```python
from build123d import *

# Parameters (mm, degrees)
ESQUISSE1_R        = 3.25
ESQUISSE1_R_2      = 2
BOSS_EXTRU_1_DEPTH = 1.5
ESQUISSE2_W        = 10
ESQUISSE2_H        = 1.5
BOSS_EXTRU_2_DEPTH = 6
CONG_1_START       = -20
CONG_1_DEPTH       = 10
CONG_1_START_2     = -6
CONG_1_2_DEPTH     = 1.5
CONG_1_START_3     = -24.5
CONG_1_3_DEPTH     = 29


with BuildPart() as part:
    # Esquisse1 → Boss.-Extru.1 (new body)
    with BuildSketch(Plane.XY):
        with BuildLine():
            Line((0, -4.5), (-20, -4.5))
            ThreePointArc((-20, -4.5), (-24.5, 0), (-20, 4.5))
            Line((-20, 4.5), (0, 4.5))
            ThreePointArc((0, 4.5), (4.5, 0), (0, -4.5))
        make_face()
        Circle(ESQUISSE1_R, mode=Mode.SUBTRACT)
        with Locations((-20, 0)):
            Circle(ESQUISSE1_R_2, mode=Mode.SUBTRACT)
    extrude(amount=BOSS_EXTRU_1_DEPTH)

    # Esquisse2 → Boss.-Extru.2 (add)
    with BuildSketch(Plane.XY.offset(1.5)):
        with Locations((-15, -5.25)):
            Rectangle(ESQUISSE2_W, ESQUISSE2_H)
    extrude(amount=-BOSS_EXTRU_2_DEPTH)

    # Congé1: read off the stored shape, not the designer's step
    # Congé1 outline → Congé1 (add)
    with BuildSketch(Plane.YZ.offset(CONG_1_START)):
        with BuildLine():
            ThreePointArc((-4.5, -1.5), (-4.060660172, -0.439339828), (-3, 0))
            Line((-3, 0), (-4.5, 0))
            Line((-4.5, 0), (-4.5, -1.5))
        make_face()
    extrude(amount=CONG_1_DEPTH)

    # Cong_1 2 outline → Cong_1 2 (cut)
    with BuildSketch(Plane(origin=(0, 0, 0), x_dir=(1, 0, 0), z_dir=(0, 1, 0)).offset(CONG_1_START_2)):
        with BuildLine():
            ThreePointArc((-20, 3.5), (-19.707106781, 4.207106781), (-19, 4.5))
            Line((-19, 4.5), (-20, 4.5))
            Line((-20, 4.5), (-20, 3.5))
        make_face()
        with BuildLine():
            ThreePointArc((-11, 4.5), (-10.292893219, 4.207106781), (-10, 3.5))
            Line((-10, 3.5), (-10, 4.5))
            Line((-10, 4.5), (-11, 4.5))
        make_face()
    extrude(amount=CONG_1_2_DEPTH, mode=Mode.SUBTRACT)

    # Cong_1 3 outline → Cong_1 3 (cut)
    with BuildSketch(Plane.YZ.offset(CONG_1_START_3)):
        with BuildLine():
            ThreePointArc((-6, -1.5), (-5.121320344, 0.621320344), (-3, 1.5))
            Line((-3, 1.5), (-6, 1.5))
            Line((-6, 1.5), (-6, -1.5))
        make_face()
    extrude(amount=CONG_1_3_DEPTH, mode=Mode.SUBTRACT)


solid = part.part
```
Source: CAD feature listing. Evaluate the final solid. Frame: model axes, mm. A direction names the side the tool comes from. Coordinates: 2 decimals unless noted, no trailing zeros. Loops run counter-clockwise (first coordinate to the right, second up) from the corner with the lowest first, then second, coordinate; pieces in that order, holes last. Notation, with made-up numbers: (76, 83) -> (82, 83) arc R11 ccw to (82, 97) -> close; hole circle Ø2 at (77, 29.5). An arc over 180 degrees is marked (long way). One line per item, written item: value. Start each with the question number.
Q1. Mould query, pull axis Y, two halves, no side actions, for faces 3 (the face through (-2.579, -1.978, 0.74)), 4 (the face through (-15, -5, -4.5)), 5 (the face through (-15, -4.5, -3)). Classes: pulls with the +Y half, pulls with the -Y half, needs draft (parallel to the pull), parting line crosses it, or undercut.
Q2. Set-up query: faces 1 (the face through (-10, 4.5, 1)), 2 (the face through (-4.9, -4.5, 0.5)). Return all of +Z, -Z, +X, -X, +Y, -Y with unobstructed straight access to the full face (end or side cutting, diameter ignored); none if empty.
Q3. Section query B-B, the plane x = 2. Return the cut outline in (y, z), and give its area (3 significant figures).
Q4. Line query: line 1 along X through (y, z) = (1.25, 1); line 2 along Y through (x, z) = (-20, 1.1); line 3 along Y through (x, z) = (0, 1.05). Output: solid intervals per line, ascending.
Q5. Section query D-D, the plane y = -2.5. Return the cut outline in (x, z), and give its area (3 significant figures).
Q6. Section query A-A, the plane y = 0. Return the cut outline in (x, z).
Q7. Section query C-C, the plane x = -12.25. Return the cut outline in (y, z), and give its area (3 significant figures).
Q8. Contact query for flat-ended pins moving along their axis: P1, Ø1.5, axis at y = -5, z = -2.5, coming from the -X side; P2, Ø4.5, axis at x = -14, y = 1, coming from the -Z side; P3, Ø1, axis at y = 2, z = 0.5, coming from the -X side; P4, Ø3, axis at x = -20, y = 0, coming from the +Z side. Output: stop coordinate, or through.
Results:
1. face 3: undercut
1. face 4: needs draft
1. face 5: pulls with the +Y half
2. face 1: +Z, -Z, +X, -X, +Y
2. face 2: +Z, -Z, +X, -Y
3. outline: (-4.03, 0) -> (-2.56, 0) -> (-2.56, 1.5) -> (-3, 1.5) arc R3 ccw to (-4.03, 1.32) -> close; (2.56, 0) -> (4.03, 0) -> (4.03, 1.5) -> (2.56, 1.5) -> close
3. area: 4.35 mm^2
4. line 1: -24.32 to -21.56, -18.44 to -3, 3 to 4.32
4. line 2: -4.5 to -2, 2 to 4.5
4. line 3: -4.5 to -3.25, 3.25 to 4.5
5. outline: (-23.74, 0) -> (-2.08, 0) -> (-2.08, 1.5) -> (-23.74, 1.5) -> close; (2.08, 0) -> (3.74, 0) -> (3.74, 1.5) -> (2.08, 1.5) -> close
5. area: 35.0 mm^2
6. outline: (-24.5, 0) -> (-22, 0) -> (-22, 1.5) -> (-24.5, 1.5) -> close; (-18, 0) -> (-3.25, 0) -> (-3.25, 1.5) -> (-18, 1.5) -> close; (3.25, 0) -> (4.5, 0) -> (4.5, 1.5) -> (3.25, 1.5) -> close
7. outline: (-6, -4.5) -> (-4.5, -4.5) -> (-4.5, -1.5) arc R1.5 cw to (-3, 0) -> (4.5, 0) -> (4.5, 1.5) -> (-3, 1.5) arc R3 ccw to (-6, -1.5) -> close
7. area: 21.1 mm^2
8. P1: x = -20
8. P2: z = 0
8. P3: x = -24.24
8. P4: through
